Input: part model. Units: mm. Frame: model coordinates. Round coordinates to 2 decimals unless told otherwise and drop trailing zeros. Loops run counter-clockwise (first coordinate to the right, second up) from the corner with the lowest first, then second, coordinate; pieces in that order, holes last. Notation, with made-up numbers: (-36.5, -7) - (-11.5, -7) arc R11 ccw to (-11.5, 13) - close; hole circle Ø4 at (9.25, -28.5). An arc over 180 degrees is marked (long way). One line per question, with ' | ' between items. Start each with the question number.
Item 1: Section A-A, the plane z = 16. Return loops of the section in (x, y).
Item 2: First-contact query: pin 1 (1.6 mm diameter, centred on x = -155.5, y = 0, fed in from -Z). Flat tip, straight axial feed; report the tip coordinate or a pass-through.
Item 3: Section B-B, the plane y = 0.1. Give the number of separate pieces and of enclosed holes in the cut face, plus the area to 3 significant figures.
Item 4: Material intervals for line 1 along X through (y, z) = (1.2, 80); line 2 along X through (y, z) = (-0.2, 55.5); line 3 along X through (y, z) = (-0.05, 73), sorted ascending.
Item 5: Draft query along Z for faces 1 (the face through (166.614, -0.022, 56.338)), 2 (the face through (158.02, 0.02, 253.02)), 3 (the face through (28, 1.588, 130)). Return one class per face: pulls with the +Z half, pulls with the -Z half, needs draft (parallel to the pull), parting line crosses it, or undercut.
```python
from build123d import *

# Parameters (mm, degrees)
SKETCH1_W               = 308.1112
SKETCH1_H               = 3.175
BOSS_EXTRUDE1_DEPTH     = 267.83
SKETCH3_W               = 155.702
SKETCH3_H               = 3.175
BOSS_EXTRUDE3_DEPTH     = 3.175
SKETCH4_W               = 50.87366
SKETCH4_H               = 3.175
BOSS_EXTRUDE4_DEPTH     = 267.83
CUT_EXTRUDE1_DEPTH      = 340.190761306
CUT_EXTRUDE3_DEPTH      = 340.190761306
SKETCH13_R              = 5
CUT_EXTRUDE4_DEPTH      = 340.190761306
LPATTERN1_COUNT         = 3
LPATTERN1_PITCH         = 12
SKETCH17_W              = 105.930619964
SKETCH17_H              = 3.175
BOSS_EXTRUDE5_DEPTH     = 3.175
SKETCH18_W              = 80
SKETCH18_H              = 3.175
BOSS_EXTRUDE6_DEPTH     = 3.175
CUT_EXTRUDE7_DEPTH      = 340.190761306
CUT_EXTRUDE7_DEPTH_BACK = 340.190761306
SKETCH25_R              = 3
CUT_EXTRUDE8_DEPTH      = 3.175
M6_CLEARANCE_HOLE1_D    = 7
M6_CLEARANCE_HOLE2_D    = 7


with BuildPart() as part:
    # Sketch1 → Boss-Extrude1 (new body)
    with BuildSketch(Plane.XY):
        Rectangle(SKETCH1_W, SKETCH1_H)
    extrude(amount=BOSS_EXTRUDE1_DEPTH)

    # Sketch3 → Boss-Extrude3 (add)
    with BuildSketch(Plane(origin=(154.0556, 0, 0), x_dir=(0, 0, -1), z_dir=(1, 0, 0))):
        with Locations((-189.979, 0)):
            Rectangle(SKETCH3_W, SKETCH3_H)
    extrude(amount=BOSS_EXTRUDE3_DEPTH)

    # Sketch4 → Boss-Extrude4 (add)
    with BuildSketch(Plane.XY.offset(267.83)):
        with Locations((182.66743, 0)):
            Rectangle(SKETCH4_W, SKETCH4_H)
    extrude(amount=-BOSS_EXTRUDE4_DEPTH)

    # Sketch6 → Cut-Extrude1 (cut, through all)
    with BuildSketch(Plane(origin=(0, 1.5875, 0), x_dir=(1, 0, 0), z_dir=(0, 1, 0))):
        Polygon((208.10426, -238.620139294), (106.50426, -267.83), (208.10426, -267.83), align=None)
    extrude(amount=-CUT_EXTRUDE1_DEPTH, mode=Mode.SUBTRACT)

    # Sketch11 → Cut-Extrude3 (cut, through all)
    with BuildSketch(Plane.XZ.offset(1.5875)):
        Polygon((-154.0556, 242.43), (-84.2056, 267.83), (-154.0556, 267.83), align=None)
    extrude(amount=-CUT_EXTRUDE3_DEPTH, mode=Mode.SUBTRACT)

    # Sketch13 → Cut-Extrude4 (cut, through all)
    with BuildSketch(Plane.XZ.offset(1.5875)):
        with Locations(Location((171.04991, 116.644763656, 0), (0, 0, 270))):
            Circle(SKETCH13_R)
        with Locations(Location((182.04991, 116.644763656, 0), (0, 0, 270))):
            Circle(SKETCH13_R)
        with Locations(Location((193.04991, 116.644763656, 0), (0, 0, 270))):
            Circle(SKETCH13_R)
        with Locations(Location((171.04991, 46.644823778, 0), (0, 0, 270))):
            Circle(SKETCH13_R)
        with Locations(Location((182.04991, 46.644823778, 0), (0, 0, 270))):
            Circle(SKETCH13_R)
        with Locations(Location((193.04991, 46.644823778, 0), (0, 0, 270))):
            Circle(SKETCH13_R)
    cut_extrude4 = extrude(amount=-CUT_EXTRUDE4_DEPTH, mode=Mode.SUBTRACT)

    # LPattern1: Cut-Extrude4 ×3
    with Locations(*[(0, 0, i * LPATTERN1_PITCH) for i in range(1, LPATTERN1_COUNT)]):
        add(cut_extrude4, mode=Mode.SUBTRACT)

    # Sketch17 → Boss-Extrude5 (add)
    with BuildSketch(Plane.ZY.offset(154.0556)):
        with Locations((189.464690018, 0)):
            Rectangle(SKETCH17_W, SKETCH17_H)
    extrude(amount=BOSS_EXTRUDE5_DEPTH)

    # Sketch18 → Boss-Extrude6 (add)
    with BuildSketch(Plane(origin=(0, 0, 0), x_dir=(-1, 0, 0), z_dir=(0, 0, -1))):
        with Locations((-2.78399998, 0)):
            Rectangle(SKETCH18_W, SKETCH18_H)
    extrude(amount=BOSS_EXTRUDE6_DEPTH)

    # Sketch23 → Cut-Extrude7 (cut, two sides: drawn at the far end of the back side and taken through both)
    with BuildSketch(Plane(origin=(0, 1.5875, 0), x_dir=(1, 0, 0), z_dir=(0, 1, 0)).offset(-CUT_EXTRUDE7_DEPTH_BACK)):
        Polygon((681.560448342, -546.290381215), (-154.0556, -242.43), (-157.2306, -241.275454545), (-992.846648342, 62.58492667), (-1600.567410773, -1608.647170014), (73.839685911, -2217.5224779), align=None)
    extrude(amount=CUT_EXTRUDE7_DEPTH + CUT_EXTRUDE7_DEPTH_BACK, mode=Mode.SUBTRACT)

    # Sketch25 → Cut-Extrude8 (cut)
    with BuildSketch(Plane.XZ.offset(1.5875)):
        with Locations(Location((-115.3206, 247.915394364, 0), (0, 0, 270))):
            Circle(SKETCH25_R)
        with Locations(Location((-50.97574, 258.94, 0), (0, 0, 270))):
            Circle(SKETCH25_R)
        with Locations(Location((11.25426, 258.94, 0), (0, 0, 270))):
            Circle(SKETCH25_R)
        with Locations(Location((73.48426, 258.94, 0), (0, 0, 270))):
            Circle(SKETCH25_R)
        with Locations(Location((172.54426, 240.761310541, 0), (0, 0, 270))):
            Circle(SKETCH25_R)
        with Locations(Location((131.90426, 252.445254824, 0), (0, 0, 270))):
            Circle(SKETCH25_R)
    extrude(amount=-CUT_EXTRUDE8_DEPTH, mode=Mode.SUBTRACT)

    # M6 Clearance Hole1 (through all)
    with Locations(Plane.XZ.offset(1.5875)):
        with Locations((180.96500002, 180.586)):
            Hole(M6_CLEARANCE_HOLE1_D / 2)

    # M6 Clearance Hole2 (through all)
    with Locations(Plane(origin=(0, -1.5875, 0), x_dir=(-1, 0, 0), z_dir=(0, -1, 0))):
        with Locations((97.77095, -212.2849914), (-3.82905, -212.2849914), (-105.42905, -212.2849914)):
            Hole(M6_CLEARANCE_HOLE2_D / 2)


solid = part.part
```
Return value:
1) outline: (-154.06, -1.59) - (154.06, -1.59) - (154.06, 1.59) - (-154.06, 1.59) - close; (157.23, -1.59) - (208.1, -1.59) - (208.1, 1.59) - (157.23, 1.59) - close
2) pin 1: z = 136.5
3) separate pieces: 1 | enclosed holes: 28 | area: 93,100 mm2
4) line 1: -154.06 to 154.06, 157.23 to 208.1 | line 2: -154.06 to 154.06, 157.23 to 167.16, 174.94 to 178.16, 185.94 to 189.16, 196.94 to 208.1 | line 3: -154.06 to 154.06, 157.23 to 166.64, 175.46 to 177.64, 186.46 to 188.64, 197.46 to 208.1
5) face 1: undercut | face 2: pulls with the +Z half | face 3: needs draft
